CAD build for the part. Positions are in the model's coordinates, mm. Face numbers are marked on the shaded views. A direction names the side the tool comes from. Give positions to 0.01 mm unless a question says otherwise; leave off trailing zeros. Write each loop counter-clockwise with the first axis right and the second up, starting at its lowest first coordinate (ties: lowest second). Pieces come first, ordered by that corner, then holes. Notation, with made-up numbers: (54, -9) -> (65, -9) arc R16 ccw to (65, 7) -> close; hole circle Ø10 at (89.5, 38). An arc over 180 degrees is marked (long way). Answer in a Markdown table with one row per item. Add a question column.
```python
from build123d import *

# Parameters (mm, degrees)
SKETCH1_R           = 17.5
BOSS_EXTRUDE1_DEPTH = 30
BOSS_EXTRUDE2_DEPTH = 7
BOSS_EXTRUDE3_DEPTH = 8


with BuildPart() as part:
    # Sketch1 → Boss-Extrude1 (new body)
    with BuildSketch(Plane.XY):
        Circle(SKETCH1_R)
        with BuildLine():
            Line((-10.583005244, 3), (-13.5, 3))
            Line((-13.5, 3), (-13.5, -3))
            Line((-13.5, -3), (-10.583005244, -3))
            ThreePointArc((-10.583005244, -3), (11, 0), (-10.583005244, 3))
        make_face(mode=Mode.SUBTRACT)
    extrude(amount=BOSS_EXTRUDE1_DEPTH)

    # Sketch2 → Boss-Extrude2 (add, symmetric)
    with BuildSketch(Plane.XY.offset(10)):
        with BuildLine():
            ThreePointArc((-2.601595129, 17.305539656), (17.451317199, 1.304426314), (0, -17.5))
            Line((0, -17.5), (99.848635444, -17.5))
            ThreePointArc((99.848635444, -17.5), (93.848635444, -15.892304845), (89.456330598, -11.5))
            Line((89.456330598, -11.5), (40.096746205, -11.5))
            ThreePointArc((40.096746205, -11.5), (23.76101461, 2.164876864), (34.325225686, 20.65764385))
            ThreePointArc((34.325225686, 20.65764385), (56.599943686, 30.676937705), (77.322925322, 43.603938264))
            ThreePointArc((77.322925322, 43.603938264), (78.075047047, 49.606129473), (81.659593785, 54.478809544))
            ThreePointArc((81.659593785, 54.478809544), (42.018242639, 30.249770758), (-2.601595129, 17.305539656))
        make_face()
    extrude(amount=BOSS_EXTRUDE2_DEPTH, both=True)

    # Sketch2_3 → Boss-Extrude3 (add, symmetric)
    with BuildSketch(Plane.XY.offset(10)):
        with BuildLine():
            ThreePointArc((99.928029407, 50.580519361), (83.802113467, 55.86775258), (78.514880248, 39.741836641))
            ThreePointArc((78.514880248, 39.741836641), (86.12549479, 18.066520063), (87.866799191, -4.84))
            ThreePointArc((87.866799191, -4.84), (99.188635444, -17.481836253), (111.830471697, -6.16))
            ThreePointArc((111.830471697, -6.16), (109.614266096, 22.993752808), (99.928029407, 50.580519361))
        make_face()
        with BuildLine():
            ThreePointArc((94.574742117, 47.870848681), (86.511784148, 50.514465291), (83.868167538, 42.451507321))
            ThreePointArc((83.868167538, 42.451507321), (91.997687616, 19.29832825), (93.857717317, -5.17))
            ThreePointArc((93.857717317, -5.17), (99.518635444, -11.490918127), (105.83955357, -5.83))
            ThreePointArc((105.83955357, -5.83), (103.74207327, 21.761944622), (94.574742117, 47.870848681))
        make_face(mode=Mode.SUBTRACT)
    extrude(amount=BOSS_EXTRUDE3_DEPTH, both=True)


solid = part.part
```
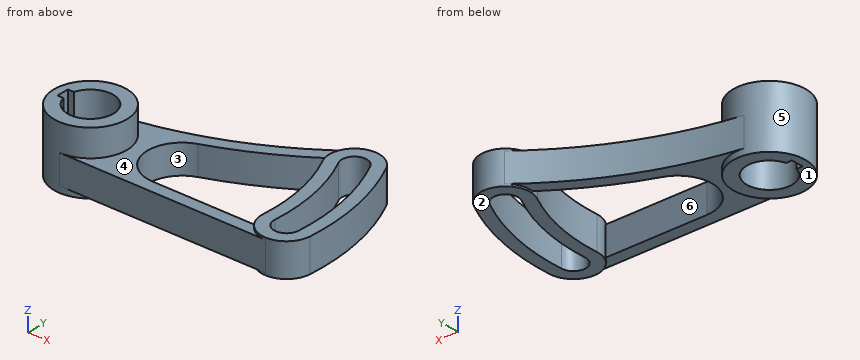
Item 1: Slice it at C-C, the plane y = 26.5. List the corners of the cut face in (x, z), then the cut area to 3 significant figures.
Item 2: Which spindle directions (+Z, -Z, +X, -X, +Y, -Y) get a long thin tool onto all of the face, cutting with end or side? Do the marked faces 1, 2 and 3. Say none if no direction does.
Item 3: Drop flat-ended pins along their axis: pin 1 Ø3 at (x, z) = (-12.5, 18.5) entering from +Y; pin 2 Ø1 at (y, z) = (38.5, 9.5) entering from +X; pin 3 Ø8 at (x, z) = (55.5, 14.5) entering from +Y; pin 4 Ø1.8 at (y, z) = (-0.5, 11) entering from +X. Give the stop position or say it passes through.
Item 4: Slice it at D-D, the plane z = 28.25. List the corners of the cut face in (x, y).
Item 5: Slice it at B-B, the plane y = 0. List the corners of the cut face in (x, z), then the cut area to 3 significant figures.
Item 6: Mould opens along Y. For the marked faces 4, 5 and 6 say: released by +Y, released by -Y, zero draft, split by the parting line, or undercut.
Item 7: Slice it at A-A, the plane x = 9. List the corners of the cut face in (y, z).
Item 8: Probe L1, parallel to Y at x = 0, z = 17.25; L2, parallel to X at y = 16, z = 5.5; L3, parallel to X at y = -1.5, z = 13.25. List the from-to ranges inside material, lowest first. Write a range as from..to.
Answer key:
| question | item | result |
|---|---|---|
| 1 | outline | (32.82, 3) -> (48.26, 3) -> (48.26, 17) -> (32.82, 17) -> close; (83.92, 2) -> (90.19, 2) -> (90.19, 18) -> (83.92, 18) -> close; (102.63, 2) -> (108.82, 2) -> (108.82, 18) -> (102.63, 18) -> close |
| 1 | area | 416 mm² |
| 2 | face 1 | -Z, +X, -X, +Y, -Y |
| 2 | face 2 | -Z, +X, +Y, -Y |
| 2 | face 3 | +Z, -Z |
| 3 | pin 1 | stops at y = 13.61 |
| 3 | pin 2 | stops at x = 105.36 |
| 3 | pin 3 | stops at y = 39.16 |
| 3 | pin 4 | stops at x = 112 |
| 4 | outline | circle Ø35 at (0, 0); hole (-13.5, -3) -> (-10.58, -3) arc R11 ccw (long way) to (-10.58, 3) -> (-13.5, 3) -> close |
| 5 | outline | (-17.5, 0) -> (-13.5, 0) -> (-13.5, 30) -> (-17.5, 30) -> close; (11, 0) -> (17.5, 0) -> (17.5, 3) -> (24.3, 3) -> (24.3, 17) -> (17.5, 17) -> (17.5, 30) -> (11, 30) -> close; (88, 2) -> (94, 2) -> (94, 18) -> (88, 18) -> close; (106, 2) -> (112, 2) -> (112, 18) -> (106, 18) -> close |
| 5 | area | 602 mm² |
| 6 | face 4 | zero draft |
| 6 | face 5 | split by the parting line |
| 6 | face 6 | undercut |
| 7 | outline | (-17.5, 3) -> (-15.01, 3) -> (-15.01, 0) -> (-6.32, 0) -> (-6.32, 30) -> (-15.01, 30) -> (-15.01, 17) -> (-17.5, 17) -> close; (6.32, 0) -> (15.01, 0) -> (15.01, 3) -> (19.45, 3) -> (19.45, 17) -> (15.01, 17) -> (15.01, 30) -> (6.32, 30) -> close |
| 8 | L1 | y = -17.5..-11, 11..17.5 |
| 8 | L2 | x = -7.09..27.58, 86.53..92.63, 104.79..110.85 |
| 8 | L3 | x = -17.44..-13.5, 10.9..24.87, 87.99..93.99, 105.99..111.99 |
